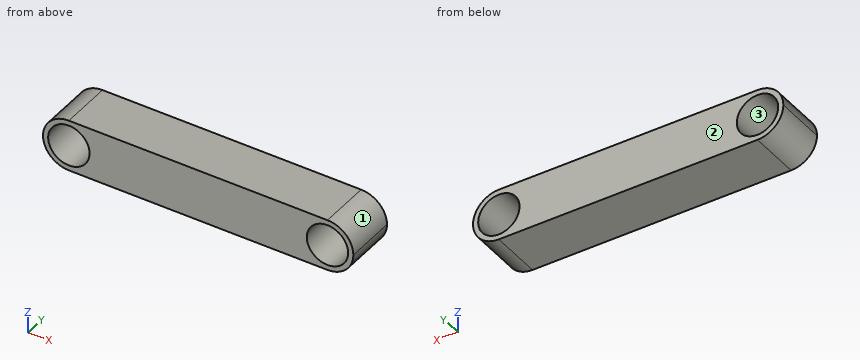
from build123d import *

# Parameters (mm, degrees)
F0_W     = 60
F0_H     = 10
F1_DEPTH = 10
F2_R     = 4
F3_DEPTH = 10.001
F4_R     = 4.99999
F5_R     = 4
F6_DEPTH = 10.001


# Not quite as in the source:
# - a fillet or chamfer is up to 0.001 mm smaller than in the source, because OpenCascade refuses the exact size


with BuildPart() as f1:
    # F0 (on Top) → F1 (new body)
    with BuildSketch(Plane.XY):
        Rectangle(F0_W, F0_H)
    extrude(amount=F1_DEPTH)

    # F2 (on face) → F3 (cut, through all)
    with BuildSketch(Plane.XZ.offset(5)):
        with Locations((-25, 5)):
            Circle(F2_R)
        with Locations((25, 5)):
            Circle(F2_R)
    extrude(amount=-F3_DEPTH, mode=Mode.SUBTRACT)

    # F4 (radius 5 in the source; OpenCascade refuses exactly that, so slightly less here)
    f4_edges = [f1.edges().sort_by_distance(p)[0] for p in [
        (-30, 0, 10),
        (-30, 0, 0),
        (30, 0, 10),
        (30, 0, 0),
    ]]
    fillet(f4_edges, radius=F4_R)

    # F5 (on face) → F6 (cut, through all)
    with BuildSketch(Plane.XZ.offset(5)):
        with Locations((45, 5)):
            Circle(F5_R)
    extrude(amount=-F6_DEPTH, mode=Mode.SUBTRACT)


solid = f1.part
The model under review builds one solid part; all positions refer to its coordinate system, in mm. Face numbers are marked on the shaded views. Coordinates: 2 decimals unless noted, no trailing zeros. Loops run counter-clockwise (first coordinate to the right, second up) from the corner with the lowest first, then second, coordinate; pieces in that order, holes last.
(1) Draft analysis for pull direction Z (two halves, no side actions). For the marked faces 1, 2 and 3, state which applies: +Z half, -Z half, draft (parallel to the pull), parting line (faces both ways), or undercut.
Determined:
face 1: +Z half
face 2: draft
face 3: undercut
(2) Consider section A-A, the plane z = 3.25. Give the boundary of the cut face in (x, y).
Determined:
outline: (-29.68, -5) - (-28.6, -5) - (-28.6, 5) - (-29.68, 5) - close; (-21.4, -5) - (21.4, -5) - (21.4, 5) - (-21.4, 5) - close; (28.6, -5) - (29.68, -5) - (29.68, 5) - (28.6, 5) - close
(3) Insertion check: P1, Ø1, axis at y = -1, z = 7, coming from the -X side. The pin has a flat end and moves straight along its axis. Give the tip position at first contact, or say it passes through.
Determined:
P1: stops at x = -29.77
(4) Consider section C-C, the plane y = 3.5. Give the number of separate pieces and of enclosed holes in the cut face, plus the area to 3 significant figures.
Determined:
separate pieces: 1
enclosed holes: 2
area: 478 mm2
(5) Consider section B-B, the plane x = -21.5. Give the boundary of the cut face in (y, z).
Determined:
outline: (-5, 0) - (5, 0) - (5, 3.06) - (-5, 3.06) - close; (-5, 6.94) - (5, 6.94) - (5, 10) - (-5, 10) - close
(6) Wall thickness on L1, parallel to X at y = -3.5, z = 5.25; L2, parallel to Z at x = -25, y = 2.75; L3, parallel to X at y = 1.5, z = 3: over which ranges is each line inside the solid? List them lowest first.
Determined:
L1: x = -29.99 to -28.99, -21.01 to 21.01, 28.99 to 29.99
L2: z = 0 to 1, 9 to 10
L3: x = -29.58 to -28.46, -21.54 to 21.54, 28.46 to 29.58
